```python
from build123d import *

# Parameters (mm, degrees)
F1_DEPTH      = 6
F2_R          = 1.5
F3_DEPTH      = 3
F3_DEPTH_BACK = 8
F4_R          = 2.99999
F5_R          = 2.99999
F6_R          = 2


# Not quite as in the source:
# - a fillet or chamfer is up to 0.001 mm smaller than in the source, because OpenCascade refuses the exact size


with BuildPart() as f1:
    # F0 (on Front) → F1 (new body)
    with BuildSketch(Plane.XZ):
        Polygon((5.5, 0), (0, 0), (0, -10), (16, -10), (16, 0), (10.5, 0), (10.5, 10), (5.5, 10), align=None)
    extrude(amount=F1_DEPTH)

    # F2 (on face) → F3 (join, two sides)
    with BuildSketch(Plane.YZ.offset(10.5)) as f3_sk:
        with Locations((-3, 6)):
            Circle(F2_R)
    extrude(amount=F3_DEPTH)
    extrude(f3_sk.sketch, amount=-F3_DEPTH_BACK)

    # F4 (radius 3 in the source; OpenCascade refuses exactly that, so slightly less here)
    f4_edges = [f1.edges().sort_by_distance(p)[0] for p in [
        (8, -6, 10),
        (8, 0, 10),
    ]]
    fillet(f4_edges, radius=F4_R)

    # F5 (radius 3 in the source; OpenCascade refuses exactly that, so slightly less here)
    f5_edges = [f1.edges().sort_by_distance(p)[0] for p in [
        (2.75, -6, 0),
        (2.75, 0, 0),
        (13.25, -6, 0),
        (13.25, 0, 0),
    ]]
    fillet(f5_edges, radius=F5_R)

    # F6
    f6_edges = [f1.edges().sort_by_distance(p)[0] for p in [
        (8, -6, -10),
        (8, 0, -10),
    ]]
    fillet(f6_edges, radius=F6_R)


solid = f1.part
```
Could you check a few things on this model? Use its own coordinates, in mm. A direction names the side the tool comes from. Give positions to 0.01 mm unless a question says otherwise; leave off trailing zeros. Order: outer loops, then holes, each group sorted by start corner. A loop starts at its lowest first (then second) coordinate and runs counter-clockwise, first axis right, second up.
Q1. I'm going to push flat-ended pins straight in: P1, Ø3, axis at y = -3.5, z = 3, coming from the +X side; P2, Ø1, axis at x = 13.5, y = -0.5, coming from the -Z side; P3, Ø3.5, axis at y = -3, z = 6, coming from the -X side. Where does each tip first touch, or does it pass through?
Q2. We'd pull the mould along Z, two halves only. Please class faces 4 (the cylindrical face through (2.71, -0.86, -0.9)), 5 (the flat face through (8, -3, -10)), 6 (the flat face through (8, 0, -2)): +Z half, -Z half, draft (parallel to the pull), parting line (faces both ways), or undercut.
Q3. For faces 1 (the cylindrical face through (4.02, -1.57, 6.45)), 2 (the cylindrical face through (11.98, -1.57, 6.45)), 3 (the flat face through (2.5, -3, 6)), which set-ups out of +Z, -Z, +X, -X, +Y, -Y let a thin tool reach every point of the face, with its end or its side?
Q4. If I drill on line 1 along X through (y, z) = (-4.3, 7.75); line 2 along Z through (x, y) = (3, -2.55); line 3 along Z through (x, y) = (4.5, -1.65), over which ranges is the centre line in solid material (lowest first)?
Q5. Suppose I cut it at D-D, the plane y = -2.35. Write out the boundary of the cut face in (x, z).
Q6. Suppose I cut it at B-B, the plane z = 6. Write out the boundary of the cut face in (x, y).
Solution:
1. P1: stops at x = 10.5
1. P2: stops at z = -9.73
1. P3: stops at x = 2.5
2. face 4: undercut
2. face 5: -Z half
2. face 6: draft
3. face 1: -X
3. face 2: +X
3. face 3: +Z, -X, +Y, -Y
4. line 1: x = 5.5 to 10.5
4. line 2: z = -10 to -0.03, 4.57 to 7.43
4. line 3: z = -9.97 to -0.32, 5.35 to 6.65
5. outline: (0, -10) - (16, -10) - (16, -0.07) - (10.5, -0.07) - (10.5, 4.65) - (13.5, 4.65) - (13.5, 7.35) - (10.5, 7.35) - (10.5, 9.93) - (5.5, 9.93) - (5.5, 7.35) - (2.5, 7.35) - (2.5, 4.65) - (5.5, 4.65) - (5.5, -0.07) - (0, -0.07) - close
6. outline: (2.5, -4.5) - (5.5, -4.5) - (5.5, -6) - (10.5, -6) - (10.5, -4.5) - (13.5, -4.5) - (13.5, -1.5) - (10.5, -1.5) - (10.5, 0) - (5.5, 0) - (5.5, -1.5) - (2.5, -1.5) - close
